Can you work these out from the drawing? Everything is in mm from the part's minimum corner. A direction names the side the tool comes from. Give positions to 0.01 mm unless a question says otherwise; leave off trailing zeros. Order: outer loops, then holes, each group sorted by start corner. A loop starts at its lowest first (then second) coordinate and runs counter-clockwise, first axis right, second up. Notation, with made-up numbers: (60.5, 63) - (116.5, 63) arc R21 cw to (116.5, 73) - close; hole circle Ø10 at (51.25, 60). An arc over 180 degrees is marked (long way). Answer as a JSON object with one key per item and string values.
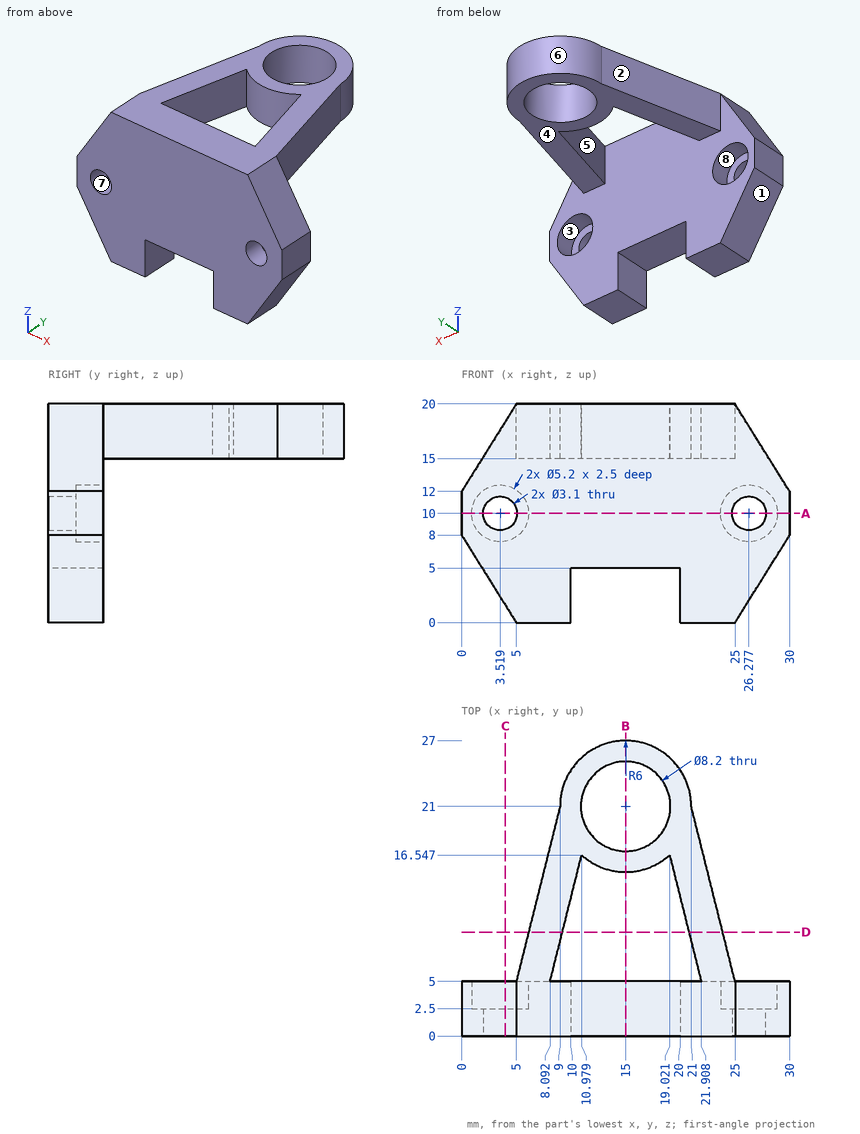
Q1. If we section it at B-B, the plane x = 15: Please give me the cut outline in (y, z).
Recorded:
{"outline": "(0, 5) - (5, 5) - (5, 20) - (0, 20) - close; (15, 15) - (16.9, 15) - (16.9, 20) - (15, 20) - close; (25.1, 15) - (27, 15) - (27, 20) - (25.1, 20) - close"}
Q2. If we section it at A-A, the plane z = 10: Please give me the cut outline in (x, y).
Recorded:
{"outline": "(0, 0) - (1.97, 0) - (1.97, 2.5) - (0.92, 2.5) - (0.92, 5) - (0, 5) - close; (5.07, 0) - (24.73, 0) - (24.73, 2.5) - (23.68, 2.5) - (23.68, 5) - (6.12, 5) - (6.12, 2.5) - (5.07, 2.5) - close; (27.83, 0) - (30, 0) - (30, 5) - (28.88, 5) - (28.88, 2.5) - (27.83, 2.5) - close"}
Q3. If we section it at D-D, the plane y = 9.5: Please give me the cut outline in (x, z) (1 decimal).
Recorded:
{"outline": "(6.1, 15) - (9.2, 15) - (9.2, 20) - (6.1, 20) - close; (20.8, 15) - (23.9, 15) - (23.9, 20) - (20.8, 20) - close"}
Q4. We'd pull the mould along Z, two halves only. Please class the marked faces 1, 2 and 3: released by +Z, released by -Z, zero draft, split by the parting line, or undercut.
Recorded:
{"face 1": "released by -Z", "face 2": "zero draft", "face 3": "undercut"}
Q5. If we section it at C-C, the plane x = 4: Please give me the cut outline in (y, z) (1 decimal).
Recorded:
{"outline": "(0, 1.6) - (5, 1.6) - (5, 7.4) - (2.5, 7.4) - (2.5, 8.5) - (0, 8.5) - close; (0, 11.5) - (2.5, 11.5) - (2.5, 12.6) - (5, 12.6) - (5, 18.4) - (0, 18.4) - close"}
Q6. I'm going to push flat-ended pins straight in: pin 1 Ø12 at (x, z) = (23, 10.5) entering from -Y; pin 2 Ø5.5 at (y, z) = (3.5, 3.5) entering from +X (1 decimal); pin 3 Ø2 at (x, z) = (12.5, 4.5) entering from +Y; pin 4 Ø3 at (x, z) = (26.28, 10) entering from -Y. Where does each tip first touch, or does it pass through?
Recorded:
{"pin 1": "stops at y = 0", "pin 2": "stops at x = 28.9", "pin 3": "stops at y = 5", "pin 4": "passes through"}
Q7. Which directions (+Z, -Z, +X, -X, +Y, -Y) give clear straight access to the entire face, cutting with the end or side of a thin tool? Please do the marked faces 4, 5, 6, 7 and 8.
Recorded:
{"face 4": "-Z, +X, -X, +Y", "face 5": "+Z, -Z", "face 6": "+Z, -Z, +Y", "face 7": "+Y, -Y", "face 8": "+Y"}
Q8. I need wall thicknesses on L1, parallel to Y at x = 15, z = 17.45; L2, parallel to Y at x = 15.75, z = 16.5; L3, parallel to X at y = 4.25, z = 11.75 (1 decimal). Which ranges of each line are inside material? Lowest first, please.
Recorded:
{"L1": "y = 0 to 5, 15 to 16.9, 25.1 to 27", "L2": "y = 0 to 5, 15.05 to 16.97, 25.03 to 26.95", "L3": "x = 0 to 1.6, 5.4 to 24.4, 28.2 to 30"}
